```python
from build123d import *

# Parameters (mm, degrees)
F1_DEPTH = 25.4
F2_DEPTH = 25.4


with BuildPart() as f1:
    # F0 (on Front) → F1 (new body)
    with BuildSketch(Plane.XZ):
        with BuildLine():
            Line((0, 0), (0, 9.525))
            ThreePointArc((0, 9.525), (-9.525, 0), (0, -9.525))
            Line((0, -9.525), (0.6773435479, -9.500885786))
            ThreePointArc((0.6773435479, -9.500885786), (6.5771572573, -6.8896028487), (9.4592491619, -1.117242271))
            ThreePointArc((9.4592491619, -1.117242271), (9.5085480823, -0.5595876752), (9.525, 0))
            Line((9.525, 0), (0, 0))
        make_face()
        with BuildLine():
            Line((0, 41.275), (0, 9.525))
            ThreePointArc((0, 9.525), (0.3388863295, 9.5189695375), (0.6773435479, 9.500885786))
            Line((0.6773435479, 9.500885786), (10.676261341, 9.1449127433))
            Line((10.676261341, 9.1449127433), (16.1720081428, 55.4634825416))
            Line((16.1720081428, 55.4634825416), (15.771858623, 58.9566822016))
            ThreePointArc((15.771858623, 58.9566822016), (15.8491936804, 58.0548119585), (15.875, 57.15))
            ThreePointArc((15.875, 57.15), (11.2253201513, 45.9246798487), (0, 41.275))
        make_face()
        with BuildLine():
            Line((0.6773435479, 9.500885786), (0, 9.525))
            Line((0, 9.525), (0, 0))
            Line((0, 0), (9.525, 0))
            ThreePointArc((9.525, 0), (6.9705567315, 6.4912990883), (0.6773435479, 9.500885786))
        make_face()
        with BuildLine():
            ThreePointArc((0.6773435479, 9.500885786), (0.3388863295, 9.5189695375), (0, 9.525))
            Line((0, 9.525), (0.6773435479, 9.500885786))
        make_face()
        with BuildLine():
            Line((0.6773435479, -9.500885786), (0, -9.525))
            ThreePointArc((0, -9.525), (0.3388863295, -9.5189695375), (0.6773435479, -9.500885786))
        make_face()
        with BuildLine():
            Line((10.676261341, 9.1449127433), (0.6773435479, 9.500885786))
            ThreePointArc((0.6773435479, 9.500885786), (6.9705567315, 6.4912990883), (9.525, 0))
            Line((9.525, 0), (9.5912078693, 0))
            Line((9.5912078693, 0), (10.676261341, 9.1449127433))
        make_face()
        with BuildLine():
            Line((0, 73.025), (0, 41.275))
            ThreePointArc((0, 41.275), (11.2253201513, 45.9246798487), (15.875, 57.15))
            ThreePointArc((15.875, 57.15), (15.8491936804, 58.0548119585), (15.771858623, 58.9566822016))
            ThreePointArc((15.771858623, 58.9566822016), (10.5672736562, 68.9968709993), (0, 73.025))
        make_face()
        with BuildLine():
            ThreePointArc((-15.7766896907, 58.9139975635), (-11.8325628315, 46.5667074197), (0, 41.275))
            Line((0, 41.275), (0, 73.025))
            ThreePointArc((0, 73.025), (-10.5832925803, 68.9825628315), (-15.7766896907, 58.9139975635))
        make_face()
        with BuildLine():
            ThreePointArc((9.4592491619, -1.117242271), (6.5771572573, -6.8896028487), (0.6773435479, -9.500885786))
            Line((0.6773435479, -9.500885786), (44.7324052746, -7.9324746146))
            ThreePointArc((44.7324052746, -7.9324746146), (38.9380895153, -5.7116327839), (36.5125, 0))
            Line((36.5125, 0), (9.5912078693, 0))
            Line((9.5912078693, 0), (9.4592491619, -1.117242271))
        make_face()
        with BuildLine():
            Line((44.7324052746, 7.9324746146), (10.676261341, 9.1449127433))
            Line((10.676261341, 9.1449127433), (9.5912078693, 0))
            Line((9.5912078693, 0), (36.5125, 0))
            ThreePointArc((36.5125, 0), (38.9380895153, 5.7116327839), (44.7324052746, 7.9324746146))
        make_face()
        with BuildLine():
            Line((-9.4751940083, 115.2727916044), (-15.7766896907, 58.9139975635))
            ThreePointArc((-15.7766896907, 58.9139975635), (-10.5832925803, 68.9825628315), (0, 73.025))
            Line((0, 73.025), (0, 104.775))
            ThreePointArc((0, 104.775), (-7.0707660487, 107.9180024691), (-9.4751940083, 115.2727916044))
        make_face()
        with BuildLine():
            Line((0, 104.775), (0, 73.025))
            ThreePointArc((0, 73.025), (10.5672736562, 68.9968709993), (15.771858623, 58.9566822016))
            Line((15.771858623, 58.9566822016), (9.5042343668, 113.6713871614))
            ThreePointArc((9.5042343668, 113.6713871614), (6.5091507784, 107.3461103587), (0, 104.775))
        make_face()
        with BuildLine():
            ThreePointArc((36.5125, 0), (38.9380895153, -5.7116327839), (44.7324052746, -7.9324746146))
            ThreePointArc((44.7324052746, -7.9324746146), (50.1616327839, -5.5119104847), (52.3875, 0))
            ThreePointArc((52.3875, 0), (50.1616327839, 5.5119104847), (44.7324052746, 7.9324746146))
            ThreePointArc((44.7324052746, 7.9324746146), (38.9380895153, 5.7116327839), (36.5125, 0))
        make_face()
        with BuildLine():
            ThreePointArc((9.525, 114.3), (0.4870328896, 123.8125403528), (-9.4751940083, 115.2727916044))
            ThreePointArc((-9.4751940083, 115.2727916044), (-7.0707660487, 107.9180024691), (0, 104.775))
            ThreePointArc((0, 104.775), (6.5091507784, 107.3461103587), (9.5042343668, 113.6713871614))
            ThreePointArc((9.5042343668, 113.6713871614), (9.5198071762, 113.9855221342), (9.525, 114.3))
        make_face()
    extrude(amount=F1_DEPTH)

    # F0 (on Front) → F2 (join)
    with BuildSketch(Plane.XZ):
        with BuildLine():
            Line((0, 0), (0, 9.525))
            ThreePointArc((0, 9.525), (-9.525, 0), (0, -9.525))
            Line((0, -9.525), (0.6773435479, -9.500885786))
            ThreePointArc((0.6773435479, -9.500885786), (6.5771572573, -6.8896028487), (9.4592491619, -1.117242271))
            ThreePointArc((9.4592491619, -1.117242271), (9.5085480823, -0.5595876752), (9.525, 0))
            Line((9.525, 0), (0, 0))
        make_face()
        with BuildLine():
            Line((0, 41.275), (0, 9.525))
            ThreePointArc((0, 9.525), (0.3388863295, 9.5189695375), (0.6773435479, 9.500885786))
            Line((0.6773435479, 9.500885786), (10.676261341, 9.1449127433))
            Line((10.676261341, 9.1449127433), (16.1720081428, 55.4634825416))
            Line((16.1720081428, 55.4634825416), (15.771858623, 58.9566822016))
            ThreePointArc((15.771858623, 58.9566822016), (15.8491936804, 58.0548119585), (15.875, 57.15))
            ThreePointArc((15.875, 57.15), (11.2253201513, 45.9246798487), (0, 41.275))
        make_face()
        with BuildLine():
            Line((0.6773435479, 9.500885786), (0, 9.525))
            Line((0, 9.525), (0, 0))
            Line((0, 0), (9.525, 0))
            ThreePointArc((9.525, 0), (6.9705567315, 6.4912990883), (0.6773435479, 9.500885786))
        make_face()
        with BuildLine():
            ThreePointArc((0.6773435479, 9.500885786), (0.3388863295, 9.5189695375), (0, 9.525))
            Line((0, 9.525), (0.6773435479, 9.500885786))
        make_face()
        with BuildLine():
            Line((0.6773435479, -9.500885786), (0, -9.525))
            ThreePointArc((0, -9.525), (0.3388863295, -9.5189695375), (0.6773435479, -9.500885786))
        make_face()
        with BuildLine():
            Line((10.676261341, 9.1449127433), (0.6773435479, 9.500885786))
            ThreePointArc((0.6773435479, 9.500885786), (6.9705567315, 6.4912990883), (9.525, 0))
            Line((9.525, 0), (9.5912078693, 0))
            Line((9.5912078693, 0), (10.676261341, 9.1449127433))
        make_face()
        with BuildLine():
            Line((0, 73.025), (0, 41.275))
            ThreePointArc((0, 41.275), (11.2253201513, 45.9246798487), (15.875, 57.15))
            ThreePointArc((15.875, 57.15), (15.8491936804, 58.0548119585), (15.771858623, 58.9566822016))
            ThreePointArc((15.771858623, 58.9566822016), (10.5672736562, 68.9968709993), (0, 73.025))
        make_face()
        with BuildLine():
            ThreePointArc((-15.7766896907, 58.9139975635), (-11.8325628315, 46.5667074197), (0, 41.275))
            Line((0, 41.275), (0, 73.025))
            ThreePointArc((0, 73.025), (-10.5832925803, 68.9825628315), (-15.7766896907, 58.9139975635))
        make_face()
        with BuildLine():
            ThreePointArc((9.4592491619, -1.117242271), (6.5771572573, -6.8896028487), (0.6773435479, -9.500885786))
            Line((0.6773435479, -9.500885786), (44.7324052746, -7.9324746146))
            ThreePointArc((44.7324052746, -7.9324746146), (38.9380895153, -5.7116327839), (36.5125, 0))
            Line((36.5125, 0), (9.5912078693, 0))
            Line((9.5912078693, 0), (9.4592491619, -1.117242271))
        make_face()
        with BuildLine():
            Line((44.7324052746, 7.9324746146), (10.676261341, 9.1449127433))
            Line((10.676261341, 9.1449127433), (9.5912078693, 0))
            Line((9.5912078693, 0), (36.5125, 0))
            ThreePointArc((36.5125, 0), (38.9380895153, 5.7116327839), (44.7324052746, 7.9324746146))
        make_face()
        with BuildLine():
            Line((-9.4751940083, 115.2727916044), (-15.7766896907, 58.9139975635))
            ThreePointArc((-15.7766896907, 58.9139975635), (-10.5832925803, 68.9825628315), (0, 73.025))
            Line((0, 73.025), (0, 104.775))
            ThreePointArc((0, 104.775), (-7.0707660487, 107.9180024691), (-9.4751940083, 115.2727916044))
        make_face()
        with BuildLine():
            Line((0, 104.775), (0, 73.025))
            ThreePointArc((0, 73.025), (10.5672736562, 68.9968709993), (15.771858623, 58.9566822016))
            Line((15.771858623, 58.9566822016), (9.5042343668, 113.6713871614))
            ThreePointArc((9.5042343668, 113.6713871614), (6.5091507784, 107.3461103587), (0, 104.775))
        make_face()
        with BuildLine():
            ThreePointArc((36.5125, 0), (38.9380895153, -5.7116327839), (44.7324052746, -7.9324746146))
            ThreePointArc((44.7324052746, -7.9324746146), (50.1616327839, -5.5119104847), (52.3875, 0))
            ThreePointArc((52.3875, 0), (50.1616327839, 5.5119104847), (44.7324052746, 7.9324746146))
            ThreePointArc((44.7324052746, 7.9324746146), (38.9380895153, 5.7116327839), (36.5125, 0))
        make_face()
        with BuildLine():
            ThreePointArc((9.525, 114.3), (0.4870328896, 123.8125403528), (-9.4751940083, 115.2727916044))
            ThreePointArc((-9.4751940083, 115.2727916044), (-7.0707660487, 107.9180024691), (0, 104.775))
            ThreePointArc((0, 104.775), (6.5091507784, 107.3461103587), (9.5042343668, 113.6713871614))
            ThreePointArc((9.5042343668, 113.6713871614), (9.5198071762, 113.9855221342), (9.525, 114.3))
        make_face()
    extrude(amount=F2_DEPTH)


solid = f1.part
```
Build history of the part. All positions in model axes, mm. A direction names the side the tool comes from. Round coordinates to 2 decimals unless told otherwise and drop trailing zeros. Order: outer loops, then holes, each group sorted by start corner. A loop starts at its lowest first (then second) coordinate and runs counter-clockwise, first axis right, second up. Notation, with made-up numbers: (57, 78.25) -> (106, 78.25) arc R24 ccw to (106, 110.25) -> close; hole circle Ø2 at (18, -12.75). An arc over 180 degrees is marked (long way). Answer in a Markdown table with one row per item.
1) Band-saw the part on C-C on x = 31. Give the cut face in (y, z).
Values:
| item | result |
|---|---|
| outline | (-25.4, -8.42) -> (0, -8.42) -> (0, 8.42) -> (-25.4, 8.42) -> close |
2) Band-saw the part on B-B on z = 85. Give the cut face in (x, y), and give its area (3 significant figures).
Values:
| item | result |
|---|---|
| outline | (-12.86, -25.4) -> (12.79, -25.4) -> (12.79, 0) -> (-12.86, 0) -> close |
| area | 651 mm2 |
3) Which spindle directions (+Z, -Z, +X, -X, +Y, -Y) get a long thin tool onto all of the face, cutting with end or side? Do faces 1 (the flat face through (10, -25.4, 43)), 2 (the flat face through (0, -13, 26)), 3 (the flat face through (13.386, -12.522, 31.98)). Say none if no direction does.
Values:
| item | result |
|---|---|
| face 1 | +Z, -Z, +X, -X, -Y |
| face 2 | -X, +Y, -Y |
| face 3 | +X, +Y, -Y |
4) Pin check, flat tips, straight feed: P1, Ø12.5, axis at y = -9.5, z = 20.5, coming from the -X side; P2, Ø3, axis at y = -11.5, z = 62, coming from the -X side; P3, Ø5, axis at y = -12, z = 35, coming from the +X side. Stop position of each tip, or through.
Values:
| item | result |
|---|---|
| P1 | x = 0 |
| P2 | x = -15.6 |
| P3 | x = 14.04 |
5) Wall check: L1, parallel to Z at x = 38.5, y = -3; L2, parallel to Z at x = 48.5, y = -9.5; L3, parallel to X at y = -13.75, z = 43. Give the ranges that are in metal, low to high.
Values:
| item | result |
|---|---|
| L1 | -8.15 to 8.15 |
| L2 | -6.83 to 6.83 |
| L3 | -7.2 to 14.69 |
